Geometry: final body of the model. Coordinates: model frame, mm. A direction names the side the tool comes from. Give positions to 0.01 mm unless a question says otherwise; leave off trailing zeros. Write each loop counter-clockwise with the first axis right and the second up, starting at its lowest first coordinate (ties: lowest second). Pieces come first, ordered by that corner, then holes. Notation, with made-up numbers: (43.25, 12.25) -> (101.25, 12.25) arc R24 ccw to (101.25, 46.25) -> close; hole circle Ø11 at (35.5, -28.75). An arc over 180 degrees is marked (long way). Answer in a Markdown table with one row per item. Add a question column.
Item 1: Section query B-B on y = 181. Output: boundary loops of the cut face in (x, z).
Item 2: Draft query along X for faces 1 (the cylindrical face through (-124.88, 504.93, -5.5)), 2 (the flat face through (-1, 500, -1)), 3 (the cylindrical face through (-19.077, 5.07, 85.907)), 4 (the flat face through (2, 510, -2)). Return one class per face: +X half, -X half, draft (parallel to the pull), parting line (faces both ways), or undercut.
Item 3: Section query A-A on z = -16. Output: boundary loops of the cut face in (x, y), plus the area to 3 significant figures.
Item 4: Section query C-C on x = -46.5. Output: boundary loops of the cut face in (y, z), plus the area to 3 significant figures.
Item 5: Material intervals for probe 1 along X at (y, z) = (504, 0); probe 2 along X at (y, z) = (135.5, 0), sorted ascending. Write a range as from..to.
Item 6: Access query for faces 5 (the cylindrical face through (89.659, 258.43, -28.235)), 6 (the cylindrical face through (95.38, 246.5, -30.04)), 7 (the flat face through (-0.5, 0, 88.4)). Directions: +Z, -Z, +X, -X, +Y, -Y. A direction counts if a zero-diameter tool reaches every point of the face in a straight line with its end or side. Return the directions, or none.
Item 7: First-contact query: P1, Ø1, axis at y = 419, z = 62, coming from the +X side; P2, Ø11.5, axis at x = -30, z = 0, coming from the -Y side; P3, Ø1.5, axis at y = 455.5, z = -19, coming from the +X side; P4, Ø7, axis at x = 0, z = -30, coming from the +Y side. Flat tips, straight axial feed; report the tip coordinate or a pass-through.
```python
from build123d import *

# Parameters (mm, degrees)
CORTE_EXTRUS_O1_REACH = 512
ESBO_O2_R             = 4.5


with BuildPart() as part:
    # Esboço1 → Revolução1 (revolve)
    with BuildSketch(Plane.XY):
        Polygon((0, 510), (125, 510), (125, 500), (100, 500), (100, 0), (88, 0), (88, 10), (94, 10), (94, 500), (0, 500), align=None)
    revolve(axis=Axis((0, 0, 0), (0, 1, 0)))

    # Esboço2 → Corte-extrusão1 (cut, up to next)
    with BuildSketch(Plane(origin=(0, 510, 0), x_dir=(1, 0, 0), z_dir=(0, 1, 0)), mode=Mode.PRIVATE) as corte_extrus_o1_sk1:
        with Locations((0, 30)):
            Circle(ESBO_O2_R)
    corte_extrus_o1_tool1 = extrude(corte_extrus_o1_sk1.sketch, amount=-CORTE_EXTRUS_O1_REACH, mode=Mode.PRIVATE) & part.part
    add(corte_extrus_o1_tool1.solids().sort_by_distance((0, 510, -30))[0], mode=Mode.SUBTRACT)
    # Esboço2 → Corte-extrusão1 (cut, up to next)
    with BuildSketch(Plane(origin=(0, 510, 0), x_dir=(1, 0, 0), z_dir=(0, 1, 0)), mode=Mode.PRIVATE) as corte_extrus_o1_sk2:
        with Locations((30, 0)):
            Circle(ESBO_O2_R)
    corte_extrus_o1_tool2 = extrude(corte_extrus_o1_sk2.sketch, amount=-CORTE_EXTRUS_O1_REACH, mode=Mode.PRIVATE) & part.part
    add(corte_extrus_o1_tool2.solids().sort_by_distance((30, 510, 0))[0], mode=Mode.SUBTRACT)
    # Esboço2 → Corte-extrusão1 (cut, up to next)
    with BuildSketch(Plane(origin=(0, 510, 0), x_dir=(1, 0, 0), z_dir=(0, 1, 0)), mode=Mode.PRIVATE) as corte_extrus_o1_sk3:
        with Locations((0, -30)):
            Circle(ESBO_O2_R)
    corte_extrus_o1_tool3 = extrude(corte_extrus_o1_sk3.sketch, amount=-CORTE_EXTRUS_O1_REACH, mode=Mode.PRIVATE) & part.part
    add(corte_extrus_o1_tool3.solids().sort_by_distance((0, 510, 30))[0], mode=Mode.SUBTRACT)
    # Esboço2 → Corte-extrusão1 (cut, up to next)
    with BuildSketch(Plane(origin=(0, 510, 0), x_dir=(1, 0, 0), z_dir=(0, 1, 0)), mode=Mode.PRIVATE) as corte_extrus_o1_sk4:
        with Locations((-30, 0)):
            Circle(ESBO_O2_R)
    corte_extrus_o1_tool4 = extrude(corte_extrus_o1_sk4.sketch, amount=-CORTE_EXTRUS_O1_REACH, mode=Mode.PRIVATE) & part.part
    add(corte_extrus_o1_tool4.solids().sort_by_distance((-30, 510, 0))[0], mode=Mode.SUBTRACT)


solid = part.part
```
Findings below:
| question | item | result |
|---|---|---|
| 1 | outline | circle Ø200 at (0, 0); hole circle Ø188 at (0, 0) |
| 2 | face 1 | parting line |
| 2 | face 2 | undercut |
| 2 | face 3 | undercut |
| 2 | face 4 | draft |
| 3 | outline | (-123.97, 500) -> (-98.71, 500) -> (-98.71, 0) -> (-86.53, 0) -> (-86.53, 10) -> (-92.63, 10) -> (-92.63, 500) -> (92.63, 500) -> (92.63, 10) -> (86.53, 10) -> (86.53, 0) -> (98.71, 0) -> (98.71, 500) -> (123.97, 500) -> (123.97, 510) -> (-123.97, 510) -> close |
| 3 | area | 8,680 mm^2 |
| 4 | outline | (0, -88.53) -> (500, -88.53) -> (500, -116.03) -> (510, -116.03) -> (510, 116.03) -> (500, 116.03) -> (500, 88.53) -> (0, 88.53) -> (0, 74.71) -> (10, 74.71) -> (10, 81.69) -> (500, 81.69) -> (500, -81.69) -> (10, -81.69) -> (10, -74.71) -> (0, -74.71) -> close |
| 4 | area | 9,300 mm^2 |
| 5 | probe 1 | x = -125..-34.5, -25.5..25.5, 34.5..125 |
| 5 | probe 2 | x = -100..-94, 94..100 |
| 6 | face 5 | none |
| 6 | face 6 | -Y |
| 6 | face 7 | +Z, -Z, +X, -X, -Y |
| 7 | P1 | stops at x = 78.85 |
| 7 | P2 | stops at y = 500 |
| 7 | P3 | stops at x = 98.32 |
| 7 | P4 | passes through |
